Can you work these out from the model? Positions are in its coordinate system, mm. A direction names the side the tool comes from. Give positions to 0.01 mm unless a question says otherwise; leave off trailing zeros. Loops run counter-clockwise (first coordinate to the right, second up) from the corner with the lowest first, then second, coordinate; pieces in that order, holes last. Notation, with made-up numbers: (-9, 19) - (39, 19) arc R32 ccw to (39, 53) - close; hole circle Ø11 at (16.25, 27). An arc over 180 degrees is marked (long way). Answer as a JSON object with one key per item and string values.
```python
from build123d import *

# Parameters (mm, degrees)
F1_DEPTH = 1263.65
F3_DEPTH = 12.7


with BuildPart() as f1:
    # F0 (on Right) → F1 (new body)
    with BuildSketch(Plane.YZ):
        with BuildLine():
            Line((-12.7, 0), (0, 0))
            Line((0, 0), (0, 38.1))
            Line((0, 38.1), (127, 38.1))
            Line((127, 38.1), (127, 0))
            Line((127, 0), (139.7, 0))
            Line((139.7, 0), (139.7, 38.1))
            ThreePointArc((139.7, 38.1), (135.980256, 47.080256), (127, 50.8))
            Line((127, 50.8), (0, 50.8))
            ThreePointArc((0, 50.8), (-8.980256, 47.080256), (-12.7, 38.1))
            Line((-12.7, 38.1), (-12.7, 0))
        make_face()
    extrude(amount=-F1_DEPTH)

    # F2 (on face) → F3 (cut)
    with BuildSketch(Plane.XZ.offset(12.7)):
        with BuildLine():
            Line((-682.625, 0), (-581.025, 0))
            Line((-581.025, 0), (-581.025, 12.7))
            ThreePointArc((-581.025, 12.7), (-584.744744, 21.680256), (-593.725, 25.4))
            Line((-593.725, 25.4), (-669.925, 25.4))
            ThreePointArc((-669.925, 25.4), (-678.905256, 21.680256), (-682.625, 12.7))
            Line((-682.625, 12.7), (-682.625, 0))
        make_face()
    extrude(amount=-F3_DEPTH, mode=Mode.SUBTRACT)


solid = f1.part
```
1) I need wall thicknesses on L1, parallel to Y at x = -764.5, z = 36.5; L2, parallel to Z at x = -1196.5, y = 111; L3, parallel to Y at x = -609, z = 18. Which ranges of each line are inside material? Lowest first, please.
Check sheet entries:
{"L1": "-12.7 to 0, 127 to 139.7", "L2": "38.1 to 50.8", "L3": "127 to 139.7"}
2) Which directions (+Z, -Z, +X, -X, +Y, -Y) give clear straight access to the entire face, cutting with the end or side of a thin tool? Please do faces 1 (the flat face through (-1263.65, 62, 43)), 2 (the flat face through (-623, 127, 19)).
Check sheet entries:
{"face 1": "+Z, -Z, -X, +Y, -Y", "face 2": "-Z, +X, -X"}
3) Imagine slicing it at B-B on y = 51. Write out the boundary of the cut face in (x, z), and give its area (3 significant figures).
Check sheet entries:
{"outline": "(-1263.65, 38.1) - (0, 38.1) - (0, 50.8) - (-1263.65, 50.8) - close", "area": "16,000 mm2"}
4) Imagine slicing it at A-A on x = -219. Write out the boundary of the cut face in (y, z), and give its area (3 significant figures).
Check sheet entries:
{"outline": "(-12.7, 0) - (0, 0) - (0, 38.1) - (127, 38.1) - (127, 0) - (139.7, 0) - (139.7, 38.1) arc R12.7 ccw to (127, 50.8) - (0, 50.8) arc R12.7 ccw to (-12.7, 38.1) - close", "area": "2,830 mm2"}
5) If we mould it in two halves opening along Y, with no side actions, what happens to faces 3 (the flat face through (-623, 139.7, 19)), 4 (the flat face through (-623, 63, 38.1)), 5 (the flat face through (-623, 64, 50.8))? For each: released by +Y, released by -Y, zero draft, split by the parting line, or undercut.
Check sheet entries:
{"face 3": "released by +Y", "face 4": "undercut", "face 5": "zero draft"}
6) I'm going to push flat-ended pins straight in: P1, Ø3, axis at x = -897, y = 42, coming from the -Z side; P2, Ø6, axis at y = 104, z = 37.5, coming from the +X side. Where does each tip first touch, or does it pass through?
Check sheet entries:
{"P1": "z = 38.1", "P2": "x = 0"}
